```python
from build123d import *

# Parameters (mm, degrees)
SKETCH1_W     = 4.572
SKETCH1_H     = 1.5748
CHAMFER1_SIZE = 0.2


with BuildPart() as part:
    # Sketch1 → Revolve1 (revolve)
    with BuildSketch(Plane(origin=(0, 0, 0), x_dir=(-1, 0, 0), z_dir=(0, 0, -1)), mode=Mode.PRIVATE) as revolve1_sk:
        with Locations((-5.842, -0.7874)):
            Rectangle(SKETCH1_W, SKETCH1_H)
    revolve(revolve1_sk.sketch.rotate(Axis((0, -1.5748, 0), (0, 1, 0)), 270), axis=Axis((0, -1.5748, 0), (0, 1, 0)))

    # Chamfer1
    chamfer1_edges = [part.edges().sort_by_distance(p)[0] for p in [
        (0, 0, -3.556),
        (0, -1.5748, -3.556),
        (0, -1.5748, -8.128),
        (0, 0, -8.128),
    ]]
    chamfer(chamfer1_edges, length=CHAMFER1_SIZE)


solid = part.part
```
Check sheet for the modelled part. Datum: model origin and axes. Units: mm. Round coordinates to 2 decimals unless told otherwise and drop trailing zeros. Order: outer loops, then holes, each group sorted by start corner. A loop starts at its lowest first (then second) coordinate and runs counter-clockwise, first axis right, second up. Notation, with made-up numbers: M 35,-34.5 L 43,-34.5 A18 cw 43,-0.5 Z; hole C 34,-22 d1. An arc over 180 degrees is marked long. Answer in a Markdown table with one row per item.
(1) Section check B-B on x = 0. Record the boundary of the cut face in (y, z).
Findings:
| item | result |
|---|---|
| outline | M -1.57,-7.93 L -1.37,-8.13 L -0.2,-8.13 L 0,-7.93 L 0,-3.76 L -0.2,-3.56 L -1.37,-3.56 L -1.57,-3.76 Z; M -1.57,3.76 L -1.37,3.56 L -0.2,3.56 L 0,3.76 L 0,7.93 L -0.2,8.13 L -1.37,8.13 L -1.57,7.93 Z |
(2) Section check A-A on z = 0. Record the boundary of the cut face in (x, y).
Findings:
| item | result |
|---|---|
| outline | M -8.13,-1.37 L -7.93,-1.57 L -3.76,-1.57 L -3.56,-1.37 L -3.56,-0.2 L -3.76,0 L -7.93,0 L -8.13,-0.2 Z; M 3.56,-1.37 L 3.76,-1.57 L 7.93,-1.57 L 8.13,-1.37 L 8.13,-0.2 L 7.93,0 L 3.76,0 L 3.56,-0.2 Z |
(3) Section check C-C on y = -0.45. Record the boundary of the cut face in (x, z), plus the area to 3 significant figures.
Findings:
| item | result |
|---|---|
| outline | C 0,0 d16.26; hole C 0,0 d7.11 |
| area | 168 mm^2 |
(4) Gauge pin test, flat end, axial feed: pin 1 (5.5 mm diameter, centred on x = 0, z = 0, fed in from +Y) (1 decimal). Record the tip position at first contact, or that the pin passes through.
Findings:
| item | result |
|---|---|
| pin 1 | passes through |
(5) Material ranges on line 1 along X through (y, z) = (-0.55, 0); line 2 along X through (y, z) = (-0.3, 0.5); line 3 along X through (y, z) = (-1, 6.5), recorded low to high. Write a range as from..to.
Findings:
| item | result |
|---|---|
| line 1 | x = -8.13..-3.56, 3.56..8.13 |
| line 2 | x = -8.11..-3.52, 3.52..8.11 |
| line 3 | x = -4.88..4.88 |
(6) Draft check along Z on faces 1 (the cylindrical face through (-3.47, -0.78, -0.77)), 2 (the flat face through (-2, 0, -4)), 3 (the cylindrical face through (-7.935, -0.779, -1.762)). Enter one of: +Z half, -Z half, draft (parallel to the pull), parting line (faces both ways), or undercut.
Findings:
| item | result |
|---|---|
| face 1 | undercut |
| face 2 | draft |
| face 3 | parting line |
